Geometry: final body of the model. Coordinates: model frame, mm. Coordinates: 2 decimals unless noted, no trailing zeros. Order: outer loops, then holes, each group sorted by start corner. A loop starts at its lowest first (then second) coordinate and runs counter-clockwise, first axis right, second up. Notation, with made-up numbers: M 49.25,88 L 73.25,88 A24 ccw 73.25,110 Z; hole C -9,23 d4. An arc over 180 degrees is marked long. Use CSV: the item, a comma, the result in double quotes. Start each with the question number.
1. Section query B-B on y = -41. Return the cut outline in (x, z).
2. Section query C-C on z = 4. Return the cut outline in (x, y).
3. Pull-direction query (X, two-part tool) for faces 1 (the flat face through (63.5, -63, 13)), 2 (the flat face through (-63.5, 1, 13)), 3 (the cylindrical face through (-19.02, -11.08, 12.52)); classes: pulls with the +X half, pulls with the -X half, needs draft (parallel to the pull), parting line crosses it, or undercut.
4. Section query A-A on x = 25.4. Return the cut outline in (y, z), and give its area (3 significant figures).
5. Section query D-D on y = -12.7. Return the cut outline in (x, z).
6. Material intervals for line 1 (Y direction, x = 25.4, z = 8.5); line 2 (X direction, y = 21, z = 17.5); line 3 (X direction, y = -12.7, z = 17.5), sorted ascending.
from build123d import *

# Parameters (mm, degrees)
F2_DEPTH = 25.4
F3_DEPTH = 25.401


with BuildPart() as f2:
    # F1 (on Top) → F2 (new body)
    with BuildSketch(Plane.XY):
        with BuildLine():
            Line((63.5, 88.9), (-63.5, 88.9))
            Line((-63.5, 88.9), (-63.5, -88.9))
            Line((-63.5, -88.9), (63.5, -88.9))
            Line((63.5, -88.9), (63.5, -35.5952505992))
            ThreePointArc((63.5, -35.5952505992), (-19.05, -12.7), (63.5, 10.1952505992))
            Line((63.5, 10.1952505992), (63.5, 88.9))
        make_face()
        with BuildLine():
            Line((63.5, -35.5952505992), (63.5, 10.1952505992))
            ThreePointArc((63.5, 10.1952505992), (-19.05, -12.7), (63.5, -35.5952505992))
        make_face()
    extrude(amount=F2_DEPTH)

    # F1 (on Top) → F3 (cut, through all)
    with BuildSketch(Plane.XY):
        with BuildLine():
            Line((63.5, -35.5952505992), (63.5, 10.1952505992))
            ThreePointArc((63.5, 10.1952505992), (-19.05, -12.7), (63.5, -35.5952505992))
        make_face()
    extrude(amount=F3_DEPTH, mode=Mode.SUBTRACT)


solid = f2.part
Results list:
1,outline,"M -63.5,0 L -8.88,0 L -8.88,25.4 L -63.5,25.4 Z; M 59.68,0 L 63.5,0 L 63.5,25.4 L 59.68,25.4 Z"
2,outline,"M -63.5,-88.9 L 63.5,-88.9 L 63.5,-35.6 A44.45 cw long 63.5,10.2 L 63.5,88.9 L -63.5,88.9 Z"
3,face 1,"pulls with the +X half"
3,face 2,"pulls with the -X half"
3,face 3,"undercut"
4,outline,"M -88.9,0 L -57.15,0 L -57.15,25.4 L -88.9,25.4 Z; M 31.75,0 L 88.9,0 L 88.9,25.4 L 31.75,25.4 Z"
4,area,"2,260 mm²"
5,outline,"M -63.5,0 L -19.05,0 L -19.05,25.4 L -63.5,25.4 Z"
6,line 1,"y = -88.9 to -57.15, 31.75 to 88.9"
6,line 2,"x = -63.5 to -3.58, 54.38 to 63.5"
6,line 3,"x = -63.5 to -19.05"
